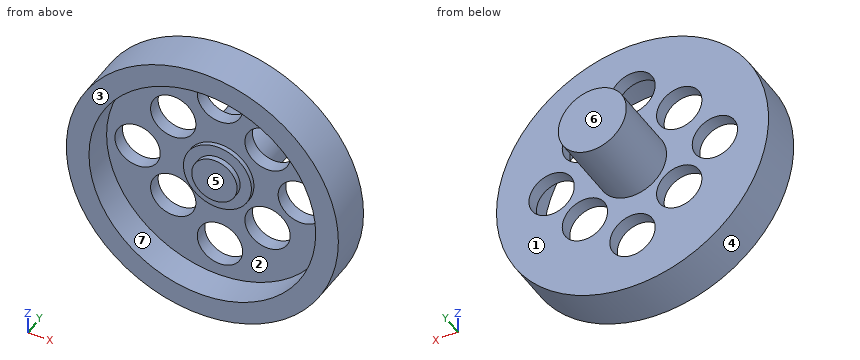
from build123d import *

# Parameters (mm, degrees)
F0_R       = 38.1
F1_DEPTH   = 12.7
F2_R       = 31.75
F3_DEPTH   = 45.466
F4_R       = 34.925
F5_DEPTH   = 3.81
F6_R       = 6.35
F7_DEPTH   = 38.354
F8_R       = 6.35
F9_DEPTH   = 26.924
F10_R      = 9.525
F11_DEPTH  = 5.08
F11_FACE_R = 9.525
F12_DEPTH  = 25.4
F13_R      = 6.35
F14_DEPTH  = 6.604


with BuildPart() as f1:
    # F0 (on Front) → F1 (new body)
    with BuildSketch(Plane.XZ):
        Circle(F0_R)
    extrude(amount=F1_DEPTH)

    # F2 (on Front) → F3 (cut)
    with BuildSketch(Plane.XZ):
        Circle(F2_R)
    extrude(amount=F3_DEPTH, mode=Mode.SUBTRACT)

    # F4 (on Front) → F5 (join)
    with BuildSketch(Plane.XZ):
        Circle(F4_R)
    extrude(amount=F5_DEPTH)

    # F6 (on Front) → F7 (cut)
    with BuildSketch(Plane.XZ):
        with Locations((-13.081, 13.081)):
            Circle(F6_R)
        with Locations((13.334999, 13.081)):
            Circle(F6_R)
        with Locations((13.334999, -11.659759)):
            Circle(F6_R)
        with Locations((-13.081, -11.659759)):
            Circle(F6_R)
    extrude(amount=F7_DEPTH, mode=Mode.SUBTRACT)

    # F8 (on Front) → F9 (cut)
    with BuildSketch(Plane.XZ):
        with Locations((0, 22.920826)):
            Circle(F8_R)
        with Locations((22.654116, 0)):
            Circle(F8_R)
        with Locations((0, -21.869805)):
            Circle(F8_R)
        with Locations((-23.065884, 0)):
            Circle(F8_R)
    extrude(amount=F9_DEPTH, mode=Mode.SUBTRACT)

    # F10 (on Front) → F11 (join)
    with BuildSketch(Plane.XZ):
        Circle(F10_R)
    extrude(amount=F11_DEPTH)

    # F11_face (on face) → F12 (join)
    with BuildSketch(Plane.XZ.offset(5.08)):
        Circle(F11_FACE_R)
    extrude(amount=-F12_DEPTH)

    # F13 (on Front) → F14 (join, symmetric)
    with BuildSketch(Plane.XZ):
        Circle(F13_R)
    extrude(amount=F14_DEPTH, both=True)


solid = f1.part
The listing builds one solid part. Answer for the finished solid, in the listing's coordinates (mm). Face numbers are marked on the shaded views. A direction names the side the tool comes from. Give positions to 0.01 mm unless a question says otherwise; leave off trailing zeros. Write each loop counter-clockwise with the first axis right and the second up, starting at its lowest first coordinate (ties: lowest second). Pieces come first, ordered by that corner, then holes. Notation, with made-up numbers: (31.5, 72) - (66.5, 72) arc R20 ccw to (66.5, 89) - close; hole circle Ø5 at (-16.5, 27). An arc over 180 degrees is marked (long way). Use a Markdown table: item, result.
1. Section D-D on y = -9 is taken. Write down the section's boundary in (x, z), plus the area to 3 significant figures.
Values follow:
| item | result |
|---|---|
| outline | circle Ø76.2 at (0, 0); hole circle Ø63.5 at (0, 0) |
| area | 1,390 mm² |
2. Section B-B on x = 0 is taken. Write down the section's boundary in (y, z) (3 decimals).
Values follow:
| item | result |
|---|---|
| outline | (-12.7, -38.1) - (0, -38.1) - (0, -28.22) - (-3.81, -28.22) - (-3.81, -31.75) - (-12.7, -31.75) - close; (-12.7, 31.75) - (-3.81, 31.75) - (-3.81, 29.271) - (0, 29.271) - (0, 38.1) - (-12.7, 38.1) - close; (-6.604, -6.35) - (-5.08, -6.35) - (-5.08, -9.525) - (-3.81, -9.525) - (-3.81, -15.52) - (0, -15.52) - (0, -9.525) - (20.32, -9.525) - (20.32, 9.525) - (0, 9.525) - (0, 16.571) - (-3.81, 16.571) - (-3.81, 9.525) - (-5.08, 9.525) - (-5.08, 6.35) - (-6.604, 6.35) - close |
3. A tool of negligible diameter and unlimited length cuts with its end or side. For the marked faces 1, 2 and 3, from which of +Z, -Z, +X, -X, +Y, -Y can it reach the whole face along a straight path? Write none if from no direction.
Values follow:
| item | result |
|---|---|
| face 1 | +Y |
| face 2 | -Y |
| face 3 | +Z, -Z, +X, -X, -Y |
4. For a pull along X with two mould halves and no side action, classify the marked faces 4, 5, 6 and 7 as released by +X, released by -X, zero draft, split by the parting line, or undercut.
Values follow:
| item | result |
|---|---|
| face 4 | split by the parting line |
| face 5 | undercut |
| face 6 | zero draft |
| face 7 | undercut |
5. Section C-C on z = 27.5 is taken. Write down the section's boundary in (x, y).
Values follow:
| item | result |
|---|---|
| outline | (-26.37, -12.7) - (-15.87, -12.7) - (-15.87, -3.81) - (-4.4, -3.81) - (-4.4, 0) - (-26.37, 0) - close; (4.4, -3.81) - (15.87, -3.81) - (15.87, -12.7) - (26.37, -12.7) - (26.37, 0) - (4.4, 0) - close |
6. Find the intervals of material crossed by probe 1 along Z at (x, y) = (0, -10); probe 2 along Z at (x, y) = (2.5, -2); probe 3 along Y at (x, z) = (18.5, 27), in increasing order. Write a range as from..to.
Values follow:
| item | result |
|---|---|
| probe 1 | z = -38.1..-31.75, 31.75..38.1 |
| probe 2 | z = -38.02..-27.71, -16.03..17.08, 28.76..38.02 |
| probe 3 | y = -12.7..0 |
7. Each of these flat-tipped pins is pushed along its axis until it touches: P1, Ø21, axis at x = 0, z = 4, coming from the -Y side; P2, Ø11.5, axis at x = 0, z = 22.92, coming from the +Y side (1 decimal); P3, Ø5, axis at x = -10, z = -1.5, coming from the +Y side; P4, Ø8, axis at y = -8, z = 27, coming from the +X side. Where does it stop, or does it pass through?
Values follow:
| item | result |
|---|---|
| P1 | stops at y = -6.6 |
| P2 | passes through |
| P3 | stops at y = 20.32 |
| P4 | stops at x = 30.37 |
8. Section A-A on z = 0 is taken. Write down the section's boundary in (x, y) (3 decimals).
Values follow:
| item | result |
|---|---|
| outline | (-38.1, -12.7) - (-31.75, -12.7) - (-31.75, -3.81) - (-29.416, -3.81) - (-29.416, 0) - (-38.1, 0) - close; (-16.716, -3.81) - (-9.525, -3.81) - (-9.525, -5.08) - (-6.35, -5.08) - (-6.35, -6.604) - (6.35, -6.604) - (6.35, -5.08) - (9.525, -5.08) - (9.525, -3.81) - (16.304, -3.81) - (16.304, 0) - (9.525, 0) - (9.525, 20.32) - (-9.525, 20.32) - (-9.525, 0) - (-16.716, 0) - close; (29.004, -3.81) - (31.75, -3.81) - (31.75, -12.7) - (38.1, -12.7) - (38.1, 0) - (29.004, 0) - close |
